Check sheet for the drawn part. Datum: minimum x, y, z corner. Units: mm. A direction names the side the tool comes from. Coordinates: 2 decimals unless noted, no trailing zeros. Write each loop counter-clockwise with the first axis right and the second up, starting at its lowest first coordinate (ties: lowest second). Pieces come first, ordered by that corner, then holes. Notation, with made-up numbers: (53.25, 26.5) -> (85.25, 26.5) arc R23 cw to (85.25, 48.5) -> close; hole circle Ø10 at (55.5, -14.75). An arc over 180 degrees is marked (long way). Answer in a Markdown table with one row per item. Add a question column.
Q1. Section check C-C, the plane x = 1.85. Record the boundary of the cut face in (y, z), and give its area (3 significant figures).
Q2. Section check D-D, the plane y = 8.75. Record the boundary of the cut face in (x, z), and give its area (3 significant figures).
Q3. Gauge pin test, flat ends, axial feed: P1, Ø1, axis at y = 4.5, z = 8.5, coming from the +X side; P2, Ø1.5, axis at x = 1, y = 4.5, coming from the +Z side. Record the tip position at first contact, or that the pin passes through.
Q4. Thickness scan on line 1 (Z direction, x = 0.95, y = 5); line 2 (Z direction, x = 2.15, y = 5); line 3 (Y direction, x = 1.2, z = 8.5). Record the ranges inside material, lowest first.
Q5. Section check B-B, the plane z = 7.5. Record the boundary of the cut face in (x, y).
Q6. Tool access check on the marked faces 4 and 5. Record the directions out of +Z, -Z, +X, -X, +Y, -Y that give a thin tool (end or side, any length) a straight path to the whole face; none if there is none.
Q7. Section check A-A, the plane y = 5. Record the boundary of the cut face in (x, z), and give its area (3 significant figures).
Q8. Release check for a two-part mould opening along Y. For the marked faces 1, 2 and 3 record: pulls with the +Y half, pulls with the -Y half, needs draft (parallel to the pull), parting line crosses it, or undercut.
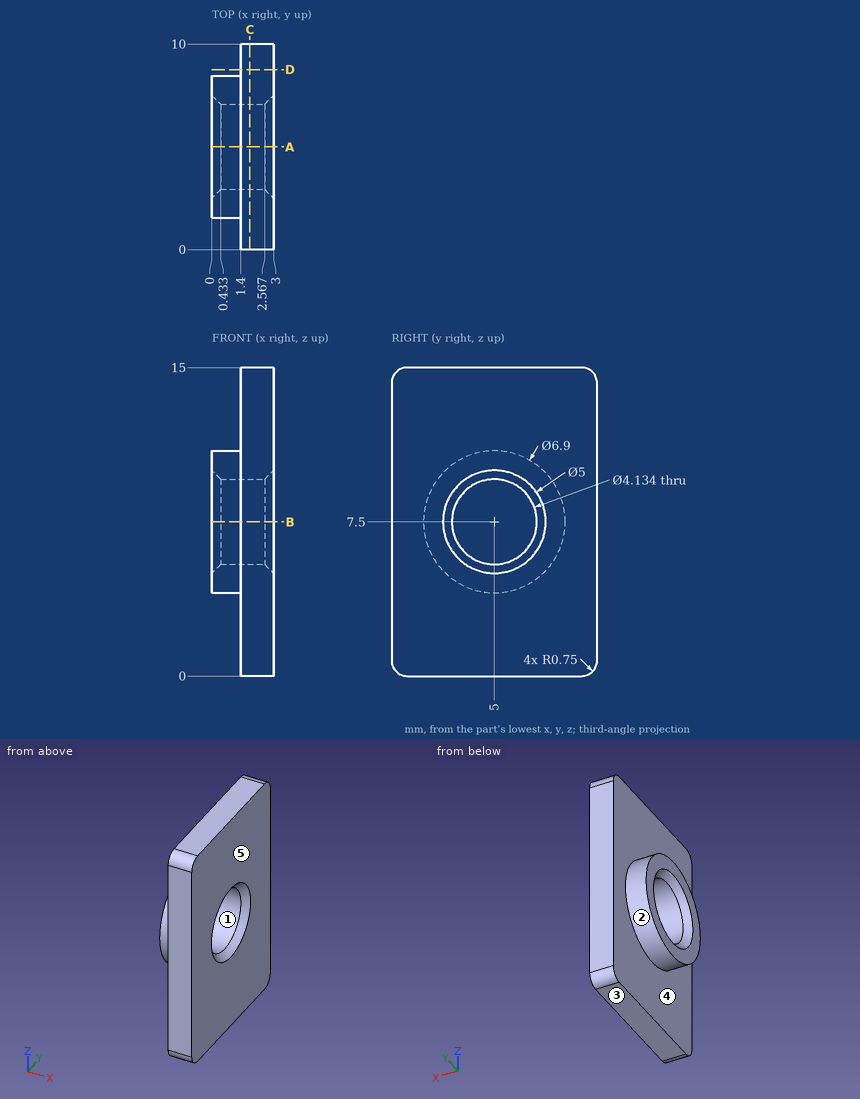
Calculated:
| question | item | result |
|---|---|---|
| 1 | outline | (0, 0.75) arc R0.75 ccw to (0.75, 0) -> (9.25, 0) arc R0.75 ccw to (10, 0.75) -> (10, 14.25) arc R0.75 ccw to (9.25, 15) -> (0.75, 15) arc R0.75 ccw to (0, 14.25) -> close; hole circle Ø4.13 at (5, 7.5) |
| 1 | area | 136 mm² |
| 2 | outline | (1.4, 0) -> (3, 0) -> (3, 15) -> (1.4, 15) -> close |
| 2 | area | 24.0 mm² |
| 3 | P1 | passes through |
| 3 | P2 | stops at z = 15 |
| 4 | line 1 | z = 4.05 to 5.43, 9.57 to 10.95 |
| 4 | line 2 | z = 0 to 5.43, 9.57 to 15 |
| 4 | line 3 | y = 1.7 to 3.19, 6.81 to 8.3 |
| 5 | outline | (0, 1.55) -> (1.4, 1.55) -> (1.4, 0) -> (3, 0) -> (3, 2.5) -> (2.57, 2.93) -> (0.43, 2.93) -> (0, 2.5) -> close; (0, 7.5) -> (0.43, 7.07) -> (2.57, 7.07) -> (3, 7.5) -> (3, 10) -> (1.4, 10) -> (1.4, 8.45) -> (0, 8.45) -> close |
| 6 | face 4 | -X |
| 6 | face 5 | +Z, -Z, +X, +Y, -Y |
| 7 | outline | (0, 4.05) -> (1.4, 4.05) -> (1.4, 0) -> (3, 0) -> (3, 5) -> (2.57, 5.43) -> (0.43, 5.43) -> (0, 5) -> close; (0, 10) -> (0.43, 9.57) -> (2.57, 9.57) -> (3, 10) -> (3, 15) -> (1.4, 15) -> (1.4, 10.95) -> (0, 10.95) -> close |
| 7 | area | 20.9 mm² |
| 8 | face 1 | undercut |
| 8 | face 2 | parting line crosses it |
| 8 | face 3 | needs draft |
